Input: part model. Units: mm. Frame: model coordinates. A direction names the side the tool comes from. Coordinates: 2 decimals unless noted, no trailing zeros. Write each loop counter-clockwise with the first axis right and the second up, starting at its lowest first coordinate (ties: lowest second). Pieces come first, ordered by that corner, then holes. Notation, with made-up numbers: (87, 11) - (133, 11) arc R7 ccw to (133, 20) - close; hole circle Ø5 at (84.5, -35.5). An arc over 180 degrees is marked (long way). One line per question, with ' | ' between items. Start each with the question number.
1) Reachability of faces 4 (the cylindrical face through (-4.032, -8.824, 7.025)), 5 (the flat face through (0, -4, 14.25)) from +Z, -Z, +X, -X, +Y, -Y: full face, straight path, thin tool, end or side. Return the list, or none.
2) First-contact query: P1, Ø1, axis at y = -6.5, z = 8.5, coming from the -X side; P2, Ø1.5, axis at x = -3.5, z = 10.5, coming from the -Y side; P3, Ø5, axis at x = 1.5, y = -7.5, coming from the -Z side. Flat tips, straight axial feed; report the tip coordinate or a pass-through.
3) Section query A-A on x = 0. Return loops of the section in (y, z), and give its area (4 significant figures).
4) Section query C-C on y = -7. Return loops of the section in (x, z), and give its area (3 significant figures).
5) Section query D-D on x = -5. Return loops of the section in (y, z).
6) Section query B-B on y = 1. Return loops of the section in (x, z).
7) Draft query along Y for faces 1 (the flat face through (-1, 6, 0)), 2 (the cylindrical face through (0.908, 9.945, -7.025)), 3 (the cylindrical face through (3, 0, 0)). Return one class per face: released by +Y, released by -Y, zero draft, split by the parting line, or undercut.
8) Line query: line 1 (Y direction, x = 0, z = 3.75); line 2 (Y direction, x = 0, z = -3.25); line 3 (Z direction, x = 4, y = -6.75). Output: solid intervals per line, ascending.
```python
from build123d import *

# Parameters (mm, degrees)
SKETCH1_R           = 7.5
BOSS_EXTRUDE1_DEPTH = 14.25
SKETCH2_R           = 7.5
BOSS_EXTRUDE2_DEPTH = 14.25
SKETCH3_R           = 3
CUT_EXTRUDE1_DEPTH  = 32.120732639


with BuildPart() as part:
    # Sketch1 → Boss-Extrude1 (new body)
    with BuildSketch(Plane.XY):
        with Locations(Location((0, -2.5, 0), (0, 0, 180))):
            Circle(SKETCH1_R)
    extrude(amount=BOSS_EXTRUDE1_DEPTH)

    # Sketch2 → Boss-Extrude2 (add)
    with BuildSketch(Plane(origin=(0, 0, 0), x_dir=(-1, 0, 0), z_dir=(0, 0, -1))):
        with Locations(Location((0, 2.5, 0), (0, 0, 199.471220634))):
            Circle(SKETCH2_R)
    extrude(amount=BOSS_EXTRUDE2_DEPTH)

    # Sketch3 → Cut-Extrude1 (cut, through all)
    with BuildSketch(Plane(origin=(0, 0, -14.25), x_dir=(-1, 0, 0), z_dir=(0, 0, -1))):
        Circle(SKETCH3_R)
    extrude(amount=-CUT_EXTRUDE1_DEPTH, mode=Mode.SUBTRACT)


solid = part.part
```
Answer key:
1) face 4: +Z | face 5: +Z, +X, -X, +Y, -Y
2) P1: x = -6.63 | P2: y = -9.48 | P3: z = 0
3) outline: (-10, 0) - (-5, 0) - (-5, -14.25) - (-3, -14.25) - (-3, 14.25) - (-10, 14.25) - close; (3, -14.25) - (10, -14.25) - (10, 0) - (5, 0) - (5, 14.25) - (3, 14.25) - close | area: 256.5 mm²
4) outline: (-6, 0) - (6, 0) - (6, 14.25) - (-6, 14.25) - close | area: 171 mm²
5) outline: (-8.09, 0) - (-3.09, 0) - (-3.09, -14.25) - (8.09, -14.25) - (8.09, 0) - (3.09, 0) - (3.09, 14.25) - (-8.09, 14.25) - close
6) outline: (-7.35, -14.25) - (-2.83, -14.25) - (-2.83, 14.25) - (-6.63, 14.25) - (-6.63, 0) - (-7.35, 0) - close; (2.83, -14.25) - (7.35, -14.25) - (7.35, 0) - (6.63, 0) - (6.63, 14.25) - (2.83, 14.25) - close
7) face 1: zero draft | face 2: split by the parting line | face 3: undercut
8) line 1: -10 to -3, 3 to 5 | line 2: -5 to -3, 3 to 10 | line 3: 0 to 14.25
